Design review of the part built by this model. Coordinates are the model's own, in mm. Coordinates: 2 decimals unless noted, no trailing zeros. Loops run counter-clockwise (first coordinate to the right, second up) from the corner with the lowest first, then second, coordinate; pieces in that order, holes last. Notation, with made-up numbers: (71.25, 33) -> (110.25, 33) arc R31 ccw to (110.25, 70) -> close; hole circle Ø6 at (56, 87.5). An arc over 180 degrees is marked (long way). Use a Markdown table: item, result. Add a question column.
Q1. Take a section at B-B on x = -26. Write out the cut boundary in (y, z).
Q2. Take a section at D-D on x = -59.1. Write out the cut boundary in (y, z).
Q3. For probe 1 along X at (y, z) = (-3.1, -16.49); probe 2 along Z at (x, y) = (-59.1, -1.9); probe 3 along Z at (x, y) = (-17, -2.15), list the stretches that pass through material, from the lowest coordinate up.
Q4. Take a section at C-C on z = -16.49. Write out the cut boundary in (x, y), plus the area to 3 significant figures.
Q5. Take a section at A-A on y = -3.35. Write out the cut boundary in (x, z).
Autodesk Fusion 360 part; units mm, degrees
sketch "Sketch1" plane through (0, 0, 0) normal (0, 1, 0) x (1, 0, 0)
  line L0 (0, 0) -> (-118.2, 0)
  line L1 (-118.2, 0) -> (-118.2, 32.98)
  line L2 (-118.2, 32.98) -> (0, 32.98)
  line L3 (0, 32.98) -> (0, 0)
  line L4 (0, 0) -> (0, 16.49)
  line L5 (-118.2, 16.49) -> (0, 16.49)
  circle A0 centre (-59.1, 16.49) radius 5.37
  point P0 (-59.1, 16.49)
  dimension "d1" = 118.2
  dimension "d2" = 32.98
  dimension "d3" = 10.74
  dimension "d4" = 59.1
sketch "Sketch2" plane through (0, 0, 0) normal (0, 1, 0) x (1, 0, 0)
  line L0 (-15.0272, 18.6866) -> (-25, 18.6866)
  arc A0 (-25, 18.6866) -> (-25, 14.6866) centre (-25, 16.6866) ccw
  line L1 (-25, 14.6866) -> (-15.0272, 14.6866)
  arc A1 (-15.0272, 14.6866) -> (-15.0272, 18.6866) centre (-15.0272, 16.6866) ccw
  line L2 (-15.0272, 16.6866) -> (-25, 16.6866) construction
  dimension "d5" = 4
extrude "Extrude1" add sketch "Sketch1" against normal blind 4 contours L0 L1 L3 L4 L5 A0 | L1 L2 L3 L5 A0
extrude "Extrude2" cut sketch "Sketch2" against normal blind 4
move_face "OffsetFaces1" offset -0.5 1 faces at (-100.29, 0, -16.49)
sketch "Sketch3" plane through (0, 0, 0) normal (0, 1, 0) x (1, 0, 0)
sketch "Sketch4" plane through (0, 0, 0) normal (0, 1, 0) x (1, 0, 0)
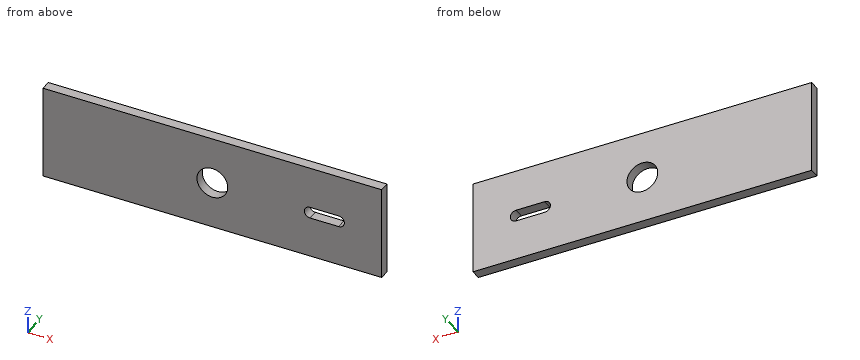
Answer list:
| question | item | result |
|---|---|---|
| 1 | outline | (-4, -32.98) -> (-0.5, -32.98) -> (-0.5, -18.42) -> (-4, -18.42) -> close; (-4, -14.95) -> (-0.5, -14.95) -> (-0.5, 0) -> (-4, 0) -> close |
| 2 | outline | (-4, -32.98) -> (-0.5, -32.98) -> (-0.5, -21.86) -> (-4, -21.86) -> close; (-4, -11.12) -> (-0.5, -11.12) -> (-0.5, 0) -> (-4, 0) -> close |
| 3 | probe 1 | -118.2 to -64.47, -53.73 to -26.99, -13.04 to 0 |
| 3 | probe 2 | -32.98 to -21.86, -11.12 to 0 |
| 3 | probe 3 | -32.98 to -18.69, -14.69 to 0 |
| 4 | outline | (-118.2, -4) -> (-64.47, -4) -> (-64.47, -0.5) -> (-118.2, -0.5) -> close; (-53.73, -4) -> (-26.99, -4) -> (-26.99, -0.5) -> (-53.73, -0.5) -> close; (-13.04, -4) -> (0, -4) -> (0, -0.5) -> (-13.04, -0.5) -> close |
| 4 | area | 327 mm² |
| 5 | outline | (-118.2, -32.98) -> (0, -32.98) -> (0, 0) -> (-118.2, 0) -> close; hole circle Ø10.74 at (-59.1, -16.49); hole (-25, -18.69) -> (-15.03, -18.69) arc R2 ccw to (-15.03, -14.69) -> (-25, -14.69) arc R2 ccw to start |
